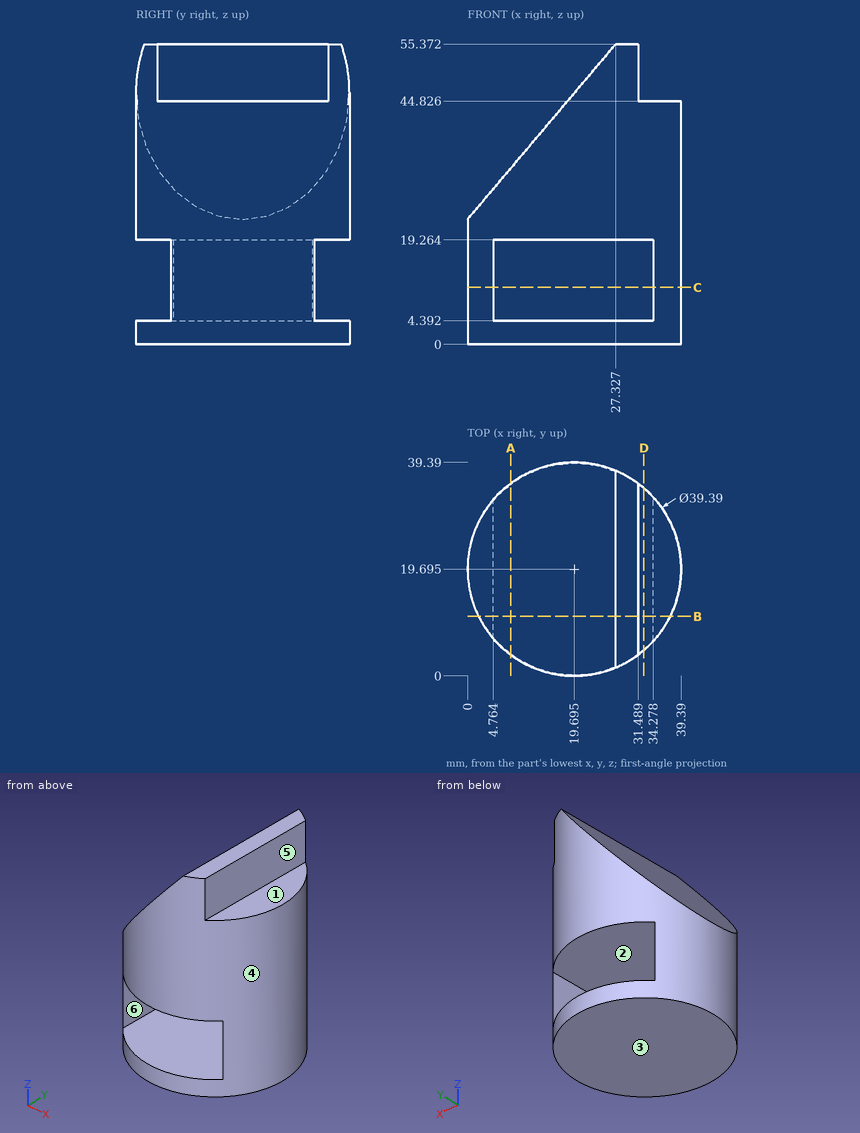
The figure shows three views and two pictorial views of one solid part (mm, origin at its lowest corner). Answer the questions. A direction names the side the tool comes from. Round coordinates to 2 decimals unless told otherwise and drop trailing zeros. Order: outer loops, then holes, each group sorted by start corner. A loop starts at its lowest first (then second) coordinate and runs counter-clockwise, first axis right, second up. Notation, with made-up numbers: M 54.5,55.5 L 80.5,55.5 A7 ccw 80.5,67.5 Z; hole C 24,17.5 d7. An arc over 180 degrees is marked long. Put each result on its own line as item: value. Start each with the question number.
Q1. Section B-B, the plane y = 11 is taken. Write down the section's boundary in (x, z), and give its area (3 significant figures).
Q2. Section A-A, the plane x = 8 is taken. Write down the section's boundary in (y, z), and give its area (3 significant figures).
Q3. Section C-C, the plane z = 10.5 is taken. Write down the section's boundary in (x, y) (1 decimal), and give its area (3 significant figures).
Q4. A tool of negligible diameter and unlimited length cuts with its end or side. For the marked faces 1, 2 and 3, from which of +Z, -Z, +X, -X, +Y, -Y can it reach the whole face along a straight path? Write none if from no direction.
Q5. For a pull along X with two mould halves and no side action, classify the marked faces 4, 5 and 6 as pulls with the +X half, pulls with the -X half, needs draft (parallel to the pull), parting line crosses it, or undercut.
Q6. Section D-D, the plane x = 32.5 is taken. Write down the section's boundary in (y, z).
Q7. Flat-ended cylindrical pins translate along their axes: pin 1 (7.5 mm diameter, centred on y = 13.5, z = 14, fed in from +X); pin 2 (5.5 mm diameter, centred on y = 15.5, z = 50.5, fed in from +X); pin 3 (4 mm diameter, centred on x = 37, y = 23.5, fed in from +Z); pin 4 (1.5 mm diameter, centred on x = 18.5, y = 8, fed in from -Z). Find the tip coordinate at first contact, or state that the pin passes through.
Q8. Straight lines are drawn through the part: L1, parallel to Z at x = 30, y = 7.5; L2, parallel to Z at x = 26, y = 23 (1 decimal); L3, parallel to Z at x = 36.5, y = 17.5. For each, find the intervals that lie inside material, in ascending order. Write a range as [from, to].
Findings below:
1. outline: M 2.02,0 L 37.37,0 L 37.37,44.83 L 31.49,44.83 L 31.49,55.37 L 27.33,55.37 L 2.02,25.43 Z; hole M 4.76,4.39 L 34.28,4.39 L 34.28,19.26 L 4.76,19.26 Z
1. area: 1,080 mm^2
2. outline: M 3.85,0 L 35.54,0 L 35.54,4.39 L 3.85,4.39 Z; M 3.85,19.26 L 35.54,19.26 L 35.54,32.5 L 3.85,32.5 Z
2. area: 559 mm^2
3. outline: M 4.8,6.9 L 4.8,32.5 A19.7 ccw Z; M 34.3,6.5 A19.7 ccw 34.3,32.9 Z
3. area: 177 mm^2
4. face 1: +Z, +X, +Y, -Y
4. face 2: +Y, -Y
4. face 3: -Z, +X, -X, +Y, -Y
5. face 4: parting line crosses it
5. face 5: pulls with the +X half
5. face 6: undercut
6. outline: M 4.73,0 L 34.66,0 L 34.66,4.39 L 4.73,4.39 Z; M 4.73,19.26 L 34.66,19.26 L 34.66,44.83 L 4.73,44.83 Z
7. pin 1: stops at x = 39.24
7. pin 2: stops at x = 31.49
7. pin 3: stops at z = 44.83
7. pin 4: stops at z = 0
8. L1: z = [0, 4.39], [19.26, 55.37]
8. L2: z = [0, 4.4], [19.3, 53.8]
8. L3: z = [0, 44.83]
